Read the model definition and answer for the solid it produces. Units are mm, in the model's axes. Give positions to 0.01 mm unless a question says otherwise; leave off trailing zeros. Order: outer loops, then holes, each group sorted by start corner. A loop starts at its lowest first (then second) coordinate and runs counter-clockwise, first axis right, second up. Notation, with made-up numbers: M 89.5,0 L 139.5,0 A26 cw 139.5,15 Z; hole C -10,-9.5 d6. An arc over 180 degrees is marked long. One line per item, written item: value. Start each with the question number.
from build123d import *

# Parameters (mm, degrees)
SKETCH1_W           = 98.782817332
SKETCH1_H           = 98.782817332
BOSS_EXTRUDE1_DEPTH = 1.000000032
SKETCH3_R           = 2.000000064
CUT_EXTRUDE2_DEPTH  = 2.000000032
SKETCH4_R           = 27.432
CUT_EXTRUDE3_DEPTH  = 2.000000032


with BuildPart() as part:
    # Sketch1 → Boss-Extrude1 (new body)
    with BuildSketch(Plane(origin=(0, 0, 0), x_dir=(1, 0, 0), z_dir=(0, 1, 0))):
        Rectangle(SKETCH1_W, SKETCH1_H)
    extrude(amount=BOSS_EXTRUDE1_DEPTH)

    # Sketch3 → Cut-Extrude2 (cut, through all)
    with BuildSketch(Plane(origin=(0, 0, 0), x_dir=(1, 0, 0), z_dir=(0, 1, 0))):
        with Locations((44.901280605, 44.901280605)):
            Circle(SKETCH3_R)
        with Locations((44.901280605, -44.901280605)):
            Circle(SKETCH3_R)
        with Locations((-44.901280605, -44.901280605)):
            Circle(SKETCH3_R)
        with Locations((-44.901280605, 44.901280605)):
            Circle(SKETCH3_R)
    extrude(amount=CUT_EXTRUDE2_DEPTH, mode=Mode.SUBTRACT)

    # Sketch4 → Cut-Extrude3 (cut, through all)
    with BuildSketch(Plane(origin=(0, 0, 0), x_dir=(1, 0, 0), z_dir=(0, 1, 0))):
        Circle(SKETCH4_R)
    extrude(amount=CUT_EXTRUDE3_DEPTH, mode=Mode.SUBTRACT)


solid = part.part
Q1. Find section C-C, the plane y = 0.65. Give the vertices of the cut face in (x, z).
Q2. Find section B-B, the plane x = 0. Give the vertices of the cut face in (y, z), then the cut area to 3 significant figures.
Q3. Consider probe 1 along Z at (x, y) = (1, 0.4); probe 2 along Z at (x, y) = (44, 0.6); probe 3 along Z at (x, y) = (14, 0.2). Determine where each line is inside the solid, lowest interval first.
Q4. Determine the mould class of faces 1 (the flat face through (21, 1, 21)), 2 (the cylindrical face through (-46.5, 0.5, 46.1)) for opening direction X: released by +X, released by -X, zero draft, split by the parting line, or undercut.
Q5. Find section A-A, the plane z = 0. Give the vertices of the cut face in (x, y), then the cut area to 3 significant figures.
Evaluation:
1. outline: M -49.39,-49.39 L 49.39,-49.39 L 49.39,49.39 L -49.39,49.39 Z; hole C -44.9,-44.9 d4; hole C -44.9,44.9 d4; hole C 0,0 d54.86; hole C 44.9,-44.9 d4; hole C 44.9,44.9 d4
2. outline: M 0,-49.39 L 1,-49.39 L 1,-27.43 L 0,-27.43 Z; M 0,27.43 L 1,27.43 L 1,49.39 L 0,49.39 Z
2. area: 43.9 mm2
3. probe 1: -49.39 to -27.41, 27.41 to 49.39
3. probe 2: -49.39 to -46.69, -43.12 to 43.12, 46.69 to 49.39
3. probe 3: -49.39 to -23.59, 23.59 to 49.39
4. face 1: zero draft
4. face 2: undercut
5. outline: M -49.39,0 L -27.43,0 L -27.43,1 L -49.39,1 Z; M 27.43,0 L 49.39,0 L 49.39,1 L 27.43,1 Z
5. area: 43.9 mm2
